The listing builds one solid part. Answer for the finished solid, in the listing's coordinates (mm). Face numbers are marked on the shaded views. Round coordinates to 2 decimals unless told otherwise and drop trailing zeros. Write each loop counter-clockwise with the first axis right and the second up, starting at its lowest first coordinate (ties: lowest second). Pieces come first, ordered by that corner, then holes.
Item 1: Find section C-C on y = -5. Give the vertices of the cut face in (x, z), then the cut area to 3 significant figures.
Item 2: Find section A-A on x = 58. Give the vertices of the cut face in (y, z), then the cut area to 3 significant figures.
Item 3: Find section D-D on z = 6. Give the vertices of the cut face in (x, y).
Item 4: Each of these flat-tipped pins is pushed along its axis until it touches: pin 1 (7 mm diameter, centred on y = -46.5, z = 25.5, fed in from -X); pin 2 (8 mm diameter, centred on x = 27, z = 3.5, fed in from -Y); pin 3 (1 mm diameter, centred on x = 57, z = 8, fed in from -Y); pin 4 (1.5 mm diameter, centred on x = 46.5, z = 15, fed in from +Y). Where does it stop, or does it pass through?
Item 5: Find the intervals of material crossed by probe 1 along Z at (x, y) = (46.5, -39.5); probe 2 along Z at (x, y) = (60, -43); probe 3 along Y at (x, z) = (55, 43), in increasing order.
Item 6: For a pull along Z with two mould halves and no side action, classify the marked faces 1, 2 and 3 as +Z half, -Z half, draft (parallel to the pull), parting line (faces both ways), or undercut.
Item 7: Find section B-B on z = 35.5. Give the vertices of the cut face in (x, y), then the cut area to 3 significant figures.
```python
from build123d import *

# Parameters (mm, degrees)
F1_DEPTH = 75
F2_W     = 46
F2_H     = 26
F3_DEPTH = 2


with BuildPart() as f1:
    # F0 (on Right) → F1 (new body)
    with BuildSketch(Plane.YZ):
        with BuildLine():
            Line((0, -2), (0, 0))
            Line((0, 0), (-48.8082464074, 0))
            ThreePointArc((-48.8082464074, 0), (-49.5742908505, 0.3572123903), (-49.7930541604, 1.1736481777))
            Line((-49.7930541604, 1.1736481777), (-41.7314827958, 46.8930912953))
            Line((-41.7314827958, 46.8930912953), (-43.7010983018, 47.2403876506))
            Line((-43.7010983018, 47.2403876506), (-52.1765613456, -0.8263518223))
            ThreePointArc((-52.1765613456, -0.8263518223), (-51.9577980357, -1.6427876097), (-51.1917535926, -2))
            Line((-51.1917535926, -2), (0, -2))
        make_face()
    extrude(amount=F1_DEPTH)

    # F2 (on face) → F3 (cut, through all)
    with BuildSketch(Plane(origin=(0, -50.4619310257, 8.8977999385), x_dir=(1, 0, 0), z_dir=(0, -0.984807753, 0.1736481777))):
        with Locations((37.5, 20.9340839315)):
            Rectangle(F2_W, F2_H)
    extrude(amount=-F3_DEPTH, mode=Mode.SUBTRACT)


solid = f1.part
```
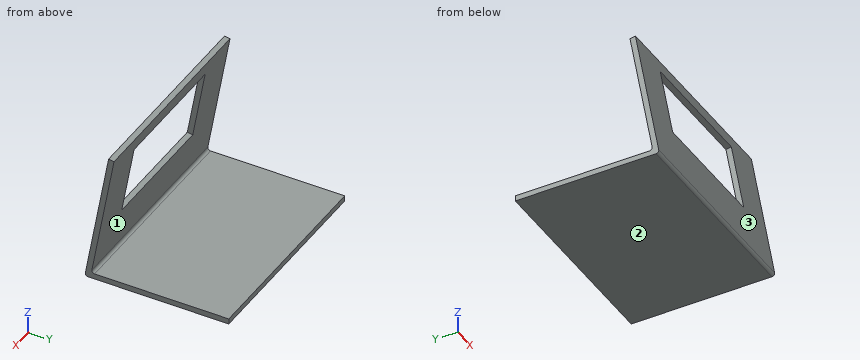
Check values:
1. outline: (0, -2) - (75, -2) - (75, 0) - (0, 0) - close
1. area: 150 mm2
2. outline: (-52.18, -0.83) arc R1 ccw to (-51.19, -2) - (0, -2) - (0, 0) - (-48.81, 0) arc R1 cw to (-49.79, 1.17) - (-47.11, 16.36) - (-49.08, 16.71) - close; (-44.57, 42.32) - (-42.6, 41.97) - (-41.73, 46.89) - (-43.7, 47.24) - close
2. area: 148 mm2
3. outline: (0, -50.97) - (75, -50.97) - (75, -48.94) - (0, -48.94) - close
4. pin 1: stops at x = 0
4. pin 2: stops at y = -52.12
4. pin 3: stops at y = -50.71
4. pin 4: stops at y = -47.22
5. probe 1: z = -2 to 0
5. probe 2: z = -2 to 0, 42.04 to 47.12
5. probe 3: y = -44.45 to -42.42
6. face 1: undercut
6. face 2: -Z half
6. face 3: +Z half
7. outline: (0, -45.77) - (14.5, -45.77) - (14.5, -43.74) - (0, -43.74) - close; (60.5, -45.77) - (75, -45.77) - (75, -43.74) - (60.5, -43.74) - close
7. area: 58.9 mm2
